Here's the drawing with two shaded views (mm, measured from the low corner). I have some questions. A direction names the side the tool comes from. Coordinates: 2 decimals unless noted, no trailing zeros. Write each loop counter-clockwise with the first axis right and the second up, starting at its lowest first coordinate (ties: lowest second). Pieces come first, ordered by that corner, then holes.
Item 1: I want a section at A-A on z = 3. Please give me the cut outline in (x, y).
Item 2: Which directions (+Z, -Z, +X, -X, +Y, -Y) give clear straight access to the entire face, cutting with the end or side of a thin tool? Please do the marked faces 1 and 2.
Item 3: I want a section at D-D on y = 2.1. Please give me the cut outline in (x, z).
Item 4: For P1, Ø1, axis at x = 10.5, z = 2, coming from the -Y side, with a flat end and sliding along its axis, tell me the tip position at first contact or that it passes through.
Item 5: Thinking about a two-plate mould opening in X: for the marked faces 3, 4, 5 and 6, which applies, +X half, -X half, draft (parallel to the pull), parting line (faces both ways), or undercut?
Item 6: If I drill on probe 1 along X at (y, z) = (2.2, 3); probe 2 along X at (y, z) = (1.35, 3); probe 3 along X at (y, z) = (0.4, 4.55), over which ranges is the centre line in solid material (lowest first)?
Item 7: I want a section at C-C on x = 15.5. Please give me the cut outline in (y, z).
Item 8: I want a section at B-B on y = 0.8. Please give me the cut outline in (x, z), then the cut area to 3 significant figures.
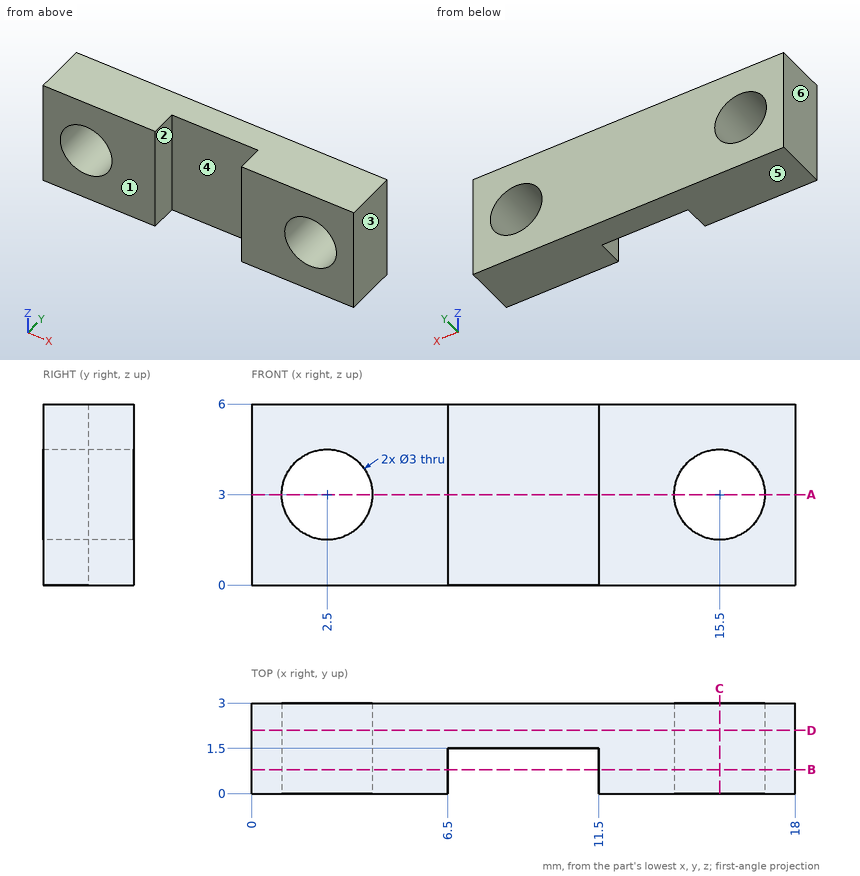
Response values:
1. outline: (0, 0) - (1, 0) - (1, 3) - (0, 3) - close; (4, 0) - (6.5, 0) - (6.5, 1.5) - (11.5, 1.5) - (11.5, 0) - (14, 0) - (14, 3) - (4, 3) - close; (17, 0) - (18, 0) - (18, 3) - (17, 3) - close
2. face 1: +Z, -Z, +X, -X, -Y
2. face 2: +Z, -Z, -Y
3. outline: (0, 0) - (18, 0) - (18, 6) - (0, 6) - close; hole circle Ø3 at (2.5, 3); hole circle Ø3 at (15.5, 3)
4. P1: stops at y = 1.5
5. face 3: +X half
5. face 4: undercut
5. face 5: draft
5. face 6: -X half
6. probe 1: x = 0 to 1, 4 to 14, 17 to 18
6. probe 2: x = 0 to 1, 4 to 6.5, 11.5 to 14, 17 to 18
6. probe 3: x = 0 to 6.5, 11.5 to 18
7. outline: (0, 0) - (3, 0) - (3, 1.5) - (0, 1.5) - close; (0, 4.5) - (3, 4.5) - (3, 6) - (0, 6) - close
8. outline: (0, 0) - (6.5, 0) - (6.5, 6) - (0, 6) - close; (11.5, 0) - (18, 0) - (18, 6) - (11.5, 6) - close; hole circle Ø3 at (2.5, 3); hole circle Ø3 at (15.5, 3)
8. area: 63.9 mm2
